```python
from build123d import *

# Parameters (mm, degrees)
SKETCH2_R                = 39
SKETCH2_R_2              = 34
BOSS_EXTRUDE1_DEPTH      = 15
SKETCH2_3_R              = 39
SKETCH2_3_R_2            = 34
SKETCH2_3_R_3            = 29
BOSS_EXTRUDE2_DEPTH      = 3
SKETCH2_4_R              = 39
SKETCH2_4_R_2            = 34
BOSS_EXTRUDE3_DEPTH      = 16
BOSS_EXTRUDE4_DEPTH      = 10
BOSS_EXTRUDE4_DEPTH_BACK = 5
SKETCH3_W                = 119
SKETCH3_H                = 10
CUT_EXTRUDE1_DEPTH       = 10
SKETCH4_R                = 1.6
CUT_EXTRUDE2_DEPTH       = 7
CUT_EXTRUDE3_DEPTH       = 27


with BuildPart() as part:
    # Sketch2 → Boss-Extrude1 (new body)
    with BuildSketch(Plane(origin=(0, 0, 0), x_dir=(1, 0, 0), z_dir=(0, 1, 0))):
        Circle(SKETCH2_R)
        Circle(SKETCH2_R_2, mode=Mode.SUBTRACT)
    extrude(amount=BOSS_EXTRUDE1_DEPTH)

    # Sketch2_3 → Boss-Extrude2 (add)
    with BuildSketch(Plane(origin=(0, 0, 0), x_dir=(1, 0, 0), z_dir=(0, 1, 0))):
        Circle(SKETCH2_3_R)
        Circle(SKETCH2_3_R_2, mode=Mode.SUBTRACT)
        Circle(SKETCH2_3_R_2)
        Circle(SKETCH2_3_R_3, mode=Mode.SUBTRACT)
    extrude(amount=-BOSS_EXTRUDE2_DEPTH)

    # Sketch2_4 → Boss-Extrude3 (add)
    with BuildSketch(Plane(origin=(0, 0, 0), x_dir=(1, 0, 0), z_dir=(0, 1, 0))):
        Circle(SKETCH2_4_R)
        Circle(SKETCH2_4_R_2, mode=Mode.SUBTRACT)
    extrude(amount=-BOSS_EXTRUDE3_DEPTH)

    # Sketch2_6 → Boss-Extrude4 (add, two sides)
    with BuildSketch(Plane(origin=(0, 0, 0), x_dir=(1, 0, 0), z_dir=(0, 1, 0))) as boss_extrude4_sk:
        with BuildLine():
            ThreePointArc((39, 0), (-27.577164466, -27.577164466), (0, 39))
            Line((0, 39), (-80, 39))
            Line((-80, 39), (-80, -80))
            Line((-80, -80), (0, -80))
            Line((0, -80), (39, -80))
            Line((39, -80), (39, 0))
        make_face()
    extrude(amount=BOSS_EXTRUDE4_DEPTH)
    extrude(boss_extrude4_sk.sketch, amount=-BOSS_EXTRUDE4_DEPTH_BACK)

    # Sketch3 → Cut-Extrude1 (cut)
    with BuildSketch(Plane(origin=(0, 10, 0), x_dir=(1, 0, 0), z_dir=(0, 1, 0))):
        with Locations((-20.5, -75)):
            Rectangle(SKETCH3_W, SKETCH3_H)
    extrude(amount=-CUT_EXTRUDE1_DEPTH, mode=Mode.SUBTRACT)

    # Sketch4 → Cut-Extrude2 (cut)
    with BuildSketch(Plane(origin=(0, 15, 0), x_dir=(1, 0, 0), z_dir=(0, 1, 0))):
        with Locations((0, 36.5)):
            Circle(SKETCH4_R)
        with Locations((25.809397513, 25.809397513)):
            Circle(SKETCH4_R)
        with Locations((36.5, 0)):
            Circle(SKETCH4_R)
        with Locations((25.809397513, -25.809397513)):
            Circle(SKETCH4_R)
        with Locations((0, -36.5)):
            Circle(SKETCH4_R)
        with Locations((-25.809397513, -25.809397513)):
            Circle(SKETCH4_R)
        with Locations((-36.5, 0)):
            Circle(SKETCH4_R)
        with Locations((-25.809397513, 25.809397513)):
            Circle(SKETCH4_R)
    extrude(amount=-CUT_EXTRUDE2_DEPTH, mode=Mode.SUBTRACT)

    # Sketch5 → Cut-Extrude3 (cut, through all)
    with BuildSketch(Plane(origin=(0, 10, 0), x_dir=(1, 0, 0), z_dir=(0, 1, 0))):
        with BuildLine():
            Line((-55.608568551, -9.603906759), (-36.513231213, -32.741929405))
            ThreePointArc((-36.513231213, -32.741929405), (-36.782743567, -35.557486737), (-39.598300899, -35.287974383))
            Line((-39.598300899, -35.287974383), (-58.693638237, -12.149951738))
            ThreePointArc((-58.693638237, -12.149951738), (-58.424125883, -9.334394405), (-55.608568551, -9.603906759))
        make_face()
    extrude(amount=-CUT_EXTRUDE3_DEPTH, mode=Mode.SUBTRACT)


solid = part.part
```
Model file for the job. Use its own axes, mm. A direction names the side the tool comes from. Round coordinates to 2 decimals unless told otherwise and drop trailing zeros. Write each loop counter-clockwise with the first axis right and the second up, starting at its lowest first coordinate (ties: lowest second). Pieces come first, ordered by that corner, then holes. Notation, with made-up numbers: (-19, 77) -> (19, 77) arc R18 cw to (19, 108) -> close; hole circle Ø1 at (79.25, -26). An arc over 180 degrees is marked (long way). Answer as CSV lines item,"result".
1. Slice it at C-C, the plane y = 6. List the corners of the cut face in (x, z).
Resolved:
outline,"(-80, -39) -> (0, -39) arc R39 ccw to (39, 0) -> (39, 70) -> (-80, 70) -> close; hole (-58.69, 12.15) arc R2 ccw to (-55.61, 9.6) -> (-36.51, 32.74) arc R2 ccw to (-39.6, 35.29) -> close; hole circle Ø68 at (0, 0)"
2. Slice it at D-D, the plane y = -8.5. List the corners of the cut face in (x, z).
Resolved:
outline,"circle Ø78 at (0, 0); hole circle Ø68 at (0, 0)"
3. Slice it at B-B, the plane x = 12.5. List the corners of the cut face in (y, z), plus the area to 3 significant figures.
Resolved:
outline,"(-16, -36.94) -> (15, -36.94) -> (15, -31.62) -> (0, -31.62) -> (0, -26.17) -> (-3, -26.17) -> (-3, -31.62) -> (-16, -31.62) -> close; (-16, 31.62) -> (-3, 31.62) -> (-3, 26.17) -> (0, 26.17) -> (0, 31.62) -> (15, 31.62) -> (15, 36.94) -> (10, 36.94) -> (10, 70) -> (0, 70) -> (0, 80) -> (-5, 80) -> (-5, 36.94) -> (-16, 36.94) -> close"
area,"909 mm²"
4. Tool access for faces 1 (the face through (39, 3, 41)), 2 (the face through (-49.012, 2.605, 23.881)), 3 (the face through (35.32, 11.55, -1.08)): list every direction of +Z, -Z, +X, -X, +Y, -Y with a clear straight run to the whole face (end or side of a thin tool).
Resolved:
face 1,"+Z, -Z, +X, +Y, -Y"
face 2,"+Y, -Y"
face 3,"+Y"
5. Drill centre lines: line 1 (Z direction, x = 0, y = 11.5); line 2 (Z direction, x = 0, y = -9); line 3 (Y direction, x = -46, z = 21). Where is each one in solid material? Low to high.
Resolved:
line 1,"-39 to -38.1, -34.9 to -34, 34 to 34.9, 38.1 to 39"
line 2,"-39 to -34, 34 to 39"
line 3,"-5 to 10"
6. Pin check, flat tips, straight feed: pin 1 Ø3 at (x, y) = (5, 7.5) entering from +Z; pin 2 Ø1.6 at (x, z) = (-37, 0) entering from +Y; pin 3 Ø6 at (x, z) = (-38, 19) entering from -Y. Stop position of each tip, or through.
Resolved:
pin 1,"z = 70"
pin 2,"y = 8"
pin 3,"y = -5"
7. Mould opens along Z. For faces 4 (the face through (-58.5, 2.6, 9.4)), 5 (the face through (-21, 5, 70)), 6 (the face through (-36.75, 2.61, 35.53)), 7 (the face through (-21, 0, 75)) say: +Z half, -Z half, draft (parallel to the pull), parting line (faces both ways), or undercut.
Resolved:
face 4,"undercut"
face 5,"+Z half"
face 6,"undercut"
face 7,"draft"
8. Slice it at A-A, the plane z = -12.5. List the corners of the cut face in (x, y).
Resolved:
outline,"(-80, -5) -> (-36.94, -5) -> (-36.94, -16) -> (-31.62, -16) -> (-31.62, -3) -> (-26.17, -3) -> (-26.17, 0) -> (-31.62, 0) -> (-31.62, 15) -> (-36.94, 15) -> (-36.94, 10) -> (-80, 10) -> close; (26.17, -3) -> (31.62, -3) -> (31.62, -16) -> (36.94, -16) -> (36.94, 15) -> (31.62, 15) -> (31.62, 0) -> (26.17, 0) -> close"
